Here's how the part is built. I have some questions about the finished solid (model axes, mm). A direction names the side the tool comes from. Round coordinates to 2 decimals unless told otherwise and drop trailing zeros. Order: outer loops, then holes, each group sorted by start corner. A loop starts at its lowest first (then second) coordinate and runs counter-clockwise, first axis right, second up. Notation, with made-up numbers: M 73,62.5 L 99,62.5 A18 ccw 99,80.5 Z; hole C -28,42 d1. An arc over 180 degrees is marked long. Use one line per item in the form item = value. Start each with the question number.
```python
from build123d import *

# Parameters (mm, degrees)
SKETCH1_R           = 3.175
BOSS_EXTRUDE1_DEPTH = 6.35
SKETCH2_R           = 2.38125
CUT_EXTRUDE2_DEPTH  = 56.721163959
FILLET1_R           = 2


with BuildPart() as part:
    # Sketch1 → Boss-Extrude1 (new body)
    with BuildSketch(Plane.XY):
        with BuildLine():
            Line((9.398, -3.7), (9.398, 28.878))
            Line((9.398, 28.878), (-9.398, 28.878))
            Line((-9.398, 28.878), (-9.398, -3.7))
            ThreePointArc((-9.398, -3.7), (-10.862466094, -7.235533906), (-14.398, -8.7))
            Line((-14.398, -8.7), (-14.398, -24.575))
            Line((-14.398, -24.575), (14.398, -24.575))
            Line((14.398, -24.575), (14.398, -8.7))
            ThreePointArc((14.398, -8.7), (10.862466094, -7.235533906), (9.398, -3.7))
        make_face()
        Circle(SKETCH1_R, mode=Mode.SUBTRACT)
        with Locations((0, 19.48)):
            Circle(SKETCH1_R, mode=Mode.SUBTRACT)
    extrude(amount=-BOSS_EXTRUDE1_DEPTH)

    # Sketch2 → Cut-Extrude2 (cut, through all)
    with BuildSketch(Plane(origin=(0, 28.878, 0), x_dir=(1, 0, 0), z_dir=(0, 1, 0))):
        with Locations(Location((5.58125, 3.175, 0), (0, 0, 270))):
            Circle(SKETCH2_R)
    extrude(amount=-CUT_EXTRUDE2_DEPTH, mode=Mode.SUBTRACT)

    # Fillet1
    # the kernel refuses this fillet: 2 mm, written as the material it takes off along each edge
    with BuildSketch(Plane(origin=(-9.398, 28.878, 5), x_dir=(1, 0, 0), z_dir=(0, 0, -1)), Plane(origin=(9.398, 28.878, 5), x_dir=(0, -1, 0), z_dir=(0, 0, -1)), Plane(origin=(-14.398, -24.575, 5), x_dir=(0, 1, 0), z_dir=(0, 0, -1))) as fillet1_piece_1:
        with BuildLine():
            CenterArc((FILLET1_R, FILLET1_R), FILLET1_R, 180, 90)
            Line((0, FILLET1_R), (0, 0))
            Line((0, 0), (FILLET1_R, 0))
        make_face()
    extrude(amount=16.35, mode=Mode.SUBTRACT)
    with BuildSketch(Plane(origin=(14.398, -8.7, 4.270509831), x_dir=(-0.9895238368781003, 0.14436958214957393, 0), z_dir=(0, 0, -1))) as fillet1_piece_2:
        with BuildLine():
            CenterArc((1.732434986, -1.979047674), FILLET1_R, 98.3007748, 73.398450401)
            Line((-0.246612688, -1.690308509), (0, 0))
            ThreePointArc((0, 0), (0.721847911, -0.052380816), (1.443695821, 0))
        make_face()
    extrude(amount=14.891019662, mode=Mode.SUBTRACT)
    with BuildSketch(Plane(origin=(14.398, -24.575, 5), x_dir=(0, 1, 0), z_dir=(0, 0, -1))) as fillet1_piece_3:
        with BuildLine():
            CenterArc((FILLET1_R, -FILLET1_R), FILLET1_R, 90, 90)
            Line((0, -FILLET1_R), (0, 0))
            Line((0, 0), (FILLET1_R, 0))
        make_face()
    extrude(amount=16.35, mode=Mode.SUBTRACT)
    with BuildSketch(Plane(origin=(-14.398, -8.7, 4.270509831), x_dir=(0.9895238368781003, 0.14436958214957393, 0), z_dir=(0, 0, -1))) as fillet1_piece_4:
        with BuildLine():
            CenterArc((1.732434986, 1.979047674), FILLET1_R, 188.300774799, 73.398450401)
            Line((-0.246612688, 1.690308509), (0, 0))
            ThreePointArc((0, 0), (0.721847911, 0.052380816), (1.443695821, 0))
        make_face()
    extrude(amount=14.891019662, mode=Mode.SUBTRACT)


solid = part.part
```
1) If we mould it in two halves opening along Y, with no side actions, what happens to faces 1 (the cylindrical face through (-13.8, -24, -3.1)), 2 (the cylindrical face through (-0.41, 22.63, -3.13)), 3 (the cylindrical face through (8.797, 28.308, -3.131))? For each: +Y half, -Y half, draft (parallel to the pull), parting line (faces both ways), or undercut.
2) On a 3-axis mill with a long thin cutter (end or side, diameter ignored), from which of +Z, -Z, +X, -X, +Y, -Y can I reach the whole of each face in a straight line? I mean faces 4 (the flat face through (9.398, 11, -3)), 5 (the flat face through (-2, 28.878, -3)), 6 (the flat face through (-9.398, 12, -3)). Say none if no direction works.
3) If we section it at A-A on x = 0: Write out the boundary of the cut face in (y, z) (3 decimals), then the cut area to 3 significant figures.
4) If I drill on line 1 (Y direction, x = 0, z = -3.75) (3 decimals); line 2 (Y direction, x = 2, z = -2) (3 decimals); line 3 (X direction, y = -2, z = -1), over which ranges is the centre line in solid material (lowest first)?
5) If we section it at B-B on z = -3: Write out the boundary of the cut face in (x, y) (3 decimals).
6) If we section it at C-C on y = 19.48: Give the number of separate pieces and of enclosed holes in the cut face, then the cut area to 3 significant figures.
7) Will these pins go through, and if not, where does the flat tip stop? pin 1 Ø12 at (x, y) = (3, -18.5) entering from +Z; pin 2 Ø2 at (y, z) = (1.5, -1) entering from -X.
Completed:
q1.face_1 = -Y half
q1.face_2 = undercut
q1.face_3 = +Y half
q2.face_4 = +Z, -Z, +X, +Y
q2.face_5 = +Z, -Z, +X, -X, +Y
q2.face_6 = +Z, -Z, -X, +Y
q3.outline = M -24.575,-6.35 L -3.175,-6.35 L -3.175,0 L -24.575,0 Z; M 3.175,-6.35 L 16.305,-6.35 L 16.305,0 L 3.175,0 Z; M 22.655,-6.35 L 28.878,-6.35 L 28.878,0 L 22.655,0 Z
q3.area = 259 mm²
q4.line_1 = -24.575 to -3.175, 3.175 to 16.305, 22.655 to 28.878
q4.line_2 = -24.575 to -2.466, 2.466 to 17.014, 21.946 to 28.878
q4.line_3 = -9.4 to -2.47, 2.47 to 4.61, 6.55 to 9.4
q5.outline = M -14.398,-22.575 A2 ccw -12.398,-24.575 L 3.206,-24.575 L 3.206,28.878 L -7.398,28.878 A2 ccw -9.398,26.878 L -9.398,-3.7 A5 cw -12.969,-8.492 A2 ccw -14.398,-10.408 Z; M 7.956,-24.575 L 12.398,-24.575 A2 ccw 14.398,-22.575 L 14.398,-10.408 A2 ccw 12.969,-8.492 A5 cw 9.398,-3.7 L 9.398,26.878 A2 ccw 7.956,28.799 Z; hole C 0,0 d6.35; hole C 0,19.48 d6.35
q6.separate_pieces = 2
q6.enclosed_holes = 1
q6.area = 61.2 mm²
q7.pin_1 = 0
q7.pin_2 = -9.4
